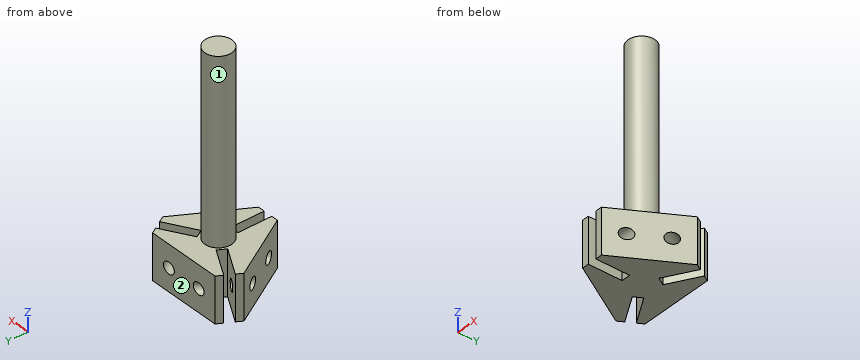
```python
from build123d import *

# Parameters (mm, degrees)
F1_DEPTH  = 20
F2_W      = 4
F2_H      = 15
F3_DEPTH  = 25
F4_R      = 6
F5_DEPTH  = 80
F6_R      = 2.5
F7_DEPTH  = 12.5
F8_R      = 2.5
F9_DEPTH  = 15
F10_R     = 2.5
F11_DEPTH = 15


with BuildPart() as f1:
    # F0 (on Top) → F1 (new body)
    with BuildSketch(Plane.XY):
        Polygon((16.5525, 15.3300930227), (-16.5525, 15.3300930227), (-21.5525, 6.6698389848), (-5, -21.9999320075), (5, -21.9999320075), (21.5525, 6.6698389848), align=None)
    extrude(amount=F1_DEPTH)

    # F2 (on face) → F3 (cut)
    with BuildSketch(Plane.XY.offset(20)):
        with Locations((0, -14.4999320075)):
            Rectangle(F2_W, F2_H)
        Polygon((20.0525, 9.2679151962), (18.0525, 12.7320168113), (5.0621189432, 5.2320168113), (7.0621189432, 1.7679151962), align=None)
        Polygon((-5.0621189432, 5.2320168113), (-18.0525, 12.7320168113), (-20.0525, 9.2679151962), (-7.0621189432, 1.7679151962), align=None)
    extrude(amount=-F3_DEPTH, mode=Mode.SUBTRACT)

    # F4 (on face) → F5 (join)
    with BuildSketch(Plane.XY.offset(20)):
        Circle(F4_R)
    extrude(amount=F5_DEPTH)

    # F6 (on Right) → F7 (cut, symmetric)
    with BuildSketch(Plane.YZ):
        with Locations((-14.4999320075, 10)):
            Circle(F6_R)
    extrude(amount=F7_DEPTH, both=True, mode=Mode.SUBTRACT)

    # F8 (on face) → F9 (cut, symmetric)
    with BuildSketch(Plane(origin=(1, 1.7320508076, 0), x_dir=(0.8660254038, -0.5, 0), z_dir=(-0.5, -0.8660254038, 0))):
        with Locations((-14.4999320075, 10)):
            Circle(F8_R)
    extrude(amount=F9_DEPTH, both=True, mode=Mode.SUBTRACT)

    # F10 (on face) → F11 (cut, symmetric)
    with BuildSketch(Plane(origin=(1, -1.7320508076, 0), x_dir=(-0.8660254038, -0.5, 0), z_dir=(-0.5, 0.8660254038, 0))):
        with Locations((-14.4999320075, 10)):
            Circle(F10_R)
    extrude(amount=F11_DEPTH, both=True, mode=Mode.SUBTRACT)


solid = f1.part
```
Work out the finished part from the listing and answer in its coordinate system (mm). Face numbers are marked on the shaded views. A direction names the side the tool comes from. Round coordinates to 2 decimals unless told otherwise and drop trailing zeros. Loops run counter-clockwise (first coordinate to the right, second up) from the corner with the lowest first, then second, coordinate; pieces in that order, holes last.
(1) The part is cut by section D-D, the plane z = 10. Give the number of separate pieces and of enclosed holes in the cut face, and give its area (3 significant figures).
Computed values:
separate pieces: 7
enclosed holes: 0
area: 691 mm2
(2) For the marked faces 1 and 2, determine the directions among +Z, -Z, +X, -X, +Y, -Y from which every point of the face is accessible in a straight line to the end or side of a thin tool.
Computed values:
face 1: +Z
face 2: +Z, -Z, +X, -X, +Y
(3) Each of these flat-tipped pins is pushed along its axis until it touches: P1, Ø1.2, axis at x = 0.5, z = 7.5, coming from the -Y side; P2, Ø12, axis at y = -17, z = 10, coming from the -X side; P3, Ø2, axis at y = 6, z = 47, coming from the +X side; P4, Ø2, axis at x = -8.5, y = 4.5, coming from the -Z side. Where does it stop, or does it pass through?
Computed values:
P1: stops at y = -7
P2: stops at x = -11.35
P3: stops at x = 3.32
P4: passes through
(4) Find the intervals of material crossed by L1, parallel to Z at x = -17, y = -1; L2, parallel to Y at x = 5.25, z = 10; L3, parallel to Y at x = 4, z = 10, in increasing order.
Computed values:
L1: z = 0 to 7.52, 12.48 to 20
L2: y = -21.57 to -17, -12 to 4.91, 5.34 to 14.91
L3: y = -22 to -17, -12 to 15.33
(5) The part is cut by section B-B, the plane y = -16. Give the vertices of the cut face in (x, z), and give its area (3 significant figures).
Computed values:
outline: (-8.46, 0) - (-2, 0) - (-2, 8) - (-8.46, 8) - close; (-8.46, 12) - (-2, 12) - (-2, 20) - (-8.46, 20) - close; (2, 0) - (8.46, 0) - (8.46, 8) - (2, 8) - close; (2, 12) - (8.46, 12) - (8.46, 20) - (2, 20) - close
area: 207 mm2
(6) The part is cut by section C-C, the plane y = -10. Give the vertices of the cut face in (x, z), and give its area (3 significant figures).
Computed values:
outline: (-11.93, 0) - (-2, 0) - (-2, 20) - (-11.93, 20) - close; (2, 0) - (11.93, 0) - (11.93, 20) - (2, 20) - close
area: 397 mm2
(7) The part is cut by section A-A, the plane x = 0. Give the vertices of the cut face in (y, z), and give its area (3 significant figures).
Computed values:
outline: (-7, 0) - (15.33, 0) - (15.33, 20) - (6, 20) - (6, 100) - (-6, 100) - (-6, 20) - (-7, 20) - close
area: 1,410 mm2
